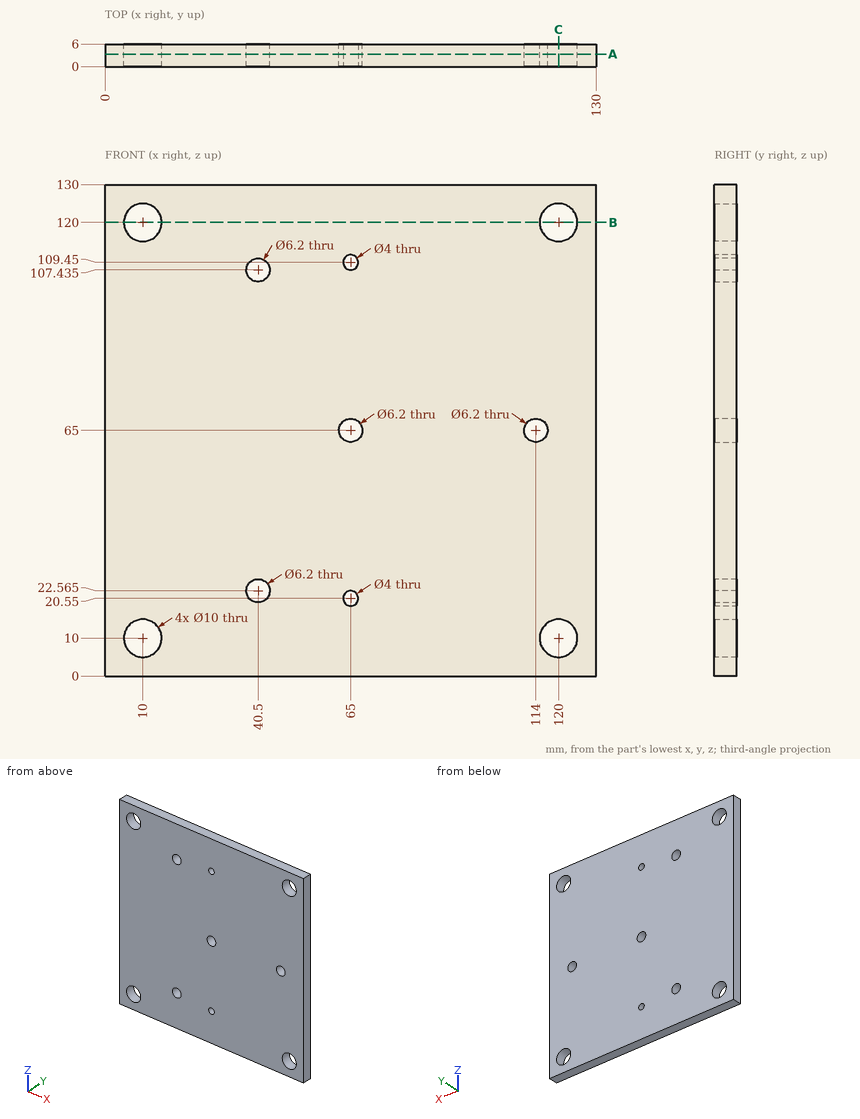
Study the drawing (mm; zero at the part's minimum x, y, z) and answer. Round coordinates to 2 decimals unless told otherwise and drop trailing zeros. Write each loop counter-clockwise with the first axis right and the second up, starting at its lowest first coordinate (ties: lowest second). Pieces come first, ordered by that corner, then holes.
1) A cutting plane is placed at C-C (x = 120). Give the vertices of the cut face in (y, z).
2) Straight lines are drawn through the part: line 1 (X direction, y = 2.15, z = 120); line 2 (Z direction, x = 65, y = 3.75). For each, find the intervals that lie inside material, in ascending order.
3) A cutting plane is placed at A-A (y = 3.35). Give the number of separate pieces and of enclosed holes in the cut face, plus the area to 3 significant figures.
4) A cutting plane is placed at B-B (z = 120). Give the vertices of the cut face in (x, y), plus the area to 3 significant figures.
5) Given pin 1 Ø7 at (x, z) = (40.5, 22.56) entering from -Y, flat-ended and moving along its own axis, determine where the tip first touches the part or whether it passes through.
Completed:
1. outline: (0, 0) - (6, 0) - (6, 5) - (0, 5) - close; (0, 15) - (6, 15) - (6, 115) - (0, 115) - close; (0, 125) - (6, 125) - (6, 130) - (0, 130) - close
2. line 1: x = 0 to 5, 15 to 115, 125 to 130
2. line 2: z = 0 to 18.55, 22.55 to 61.9, 68.1 to 107.45, 111.45 to 130
3. separate pieces: 1
3. enclosed holes: 10
3. area: 16,400 mm2
4. outline: (0, 0) - (5, 0) - (5, 6) - (0, 6) - close; (15, 0) - (115, 0) - (115, 6) - (15, 6) - close; (125, 0) - (130, 0) - (130, 6) - (125, 6) - close
4. area: 660 mm2
5. pin 1: stops at y = 0
